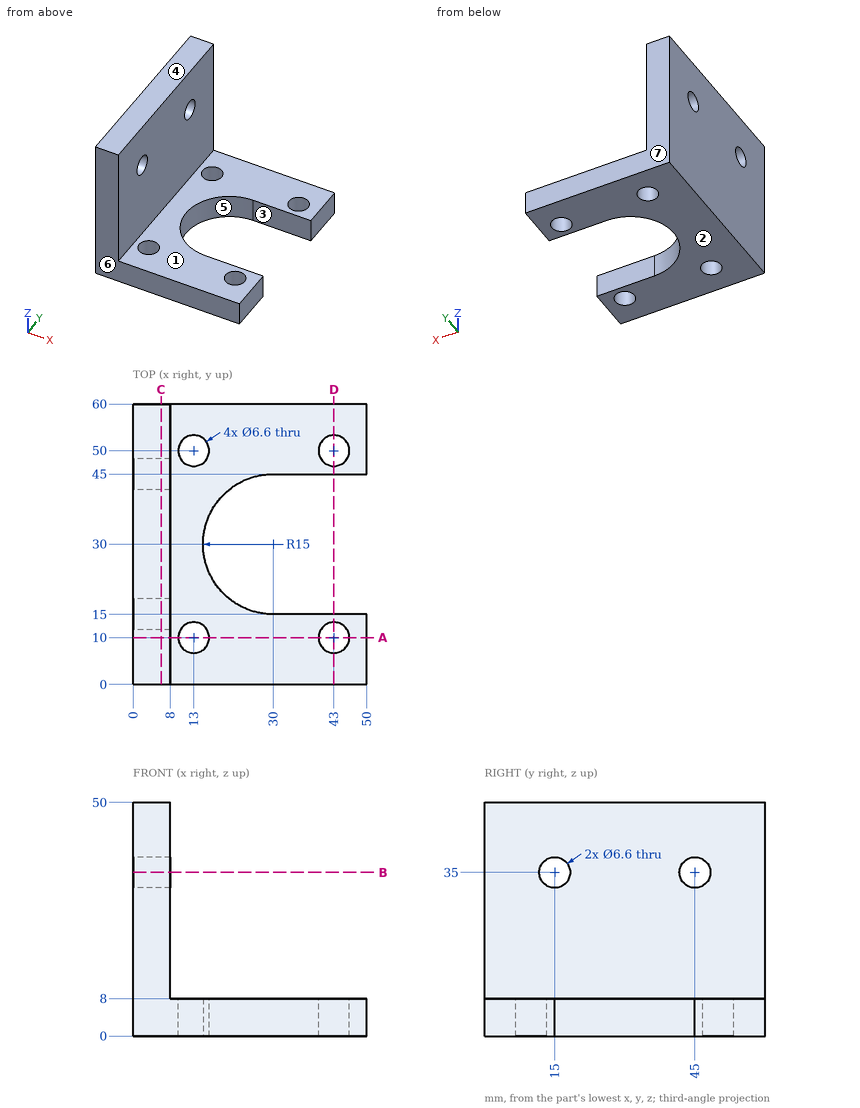
Can you work these out from the drawing? Everything is in mm from the part's minimum corner. A direction names the side the tool comes from. Round coordinates to 2 decimals unless told otherwise and drop trailing zeros. Order: outer loops, then holes, each group sorted by start corner. A loop starts at its lowest first (then second) coordinate and runs counter-clockwise, first axis right, second up. Notation, with made-up numbers: (89, 25.5) -> (129, 25.5) arc R26 ccw to (129, 58.5) -> close; hole circle Ø6 at (36, 42). An arc over 180 degrees is marked (long way). Return JSON: item names as keys, results as strings. Group by question number.
1. If we section it at C-C, the plane x = 6: Write out the boundary of the cut face in (y, z).
2. I need wall thicknesses on line 1 (Y direction, x = 13, z = 2.5); line 2 (X direction, y = 10, z = 3.75); line 3 (X direction, y = 8, z = 32.5). Which ranges of each line are inside material? Lowest first, please. Write a range as [from, to].
3. If we section it at D-D, the plane x = 43: Write out the boundary of the cut face in (y, z), then the cut area to 3 significant figures.
4. Will these pins go through, and if not, where does the flat tip stop? pin 1 (5 mm diameter, centred on y = 24.5, z = 6, fed in from +X); pin 2 (5.5 mm diameter, centred on y = 45, z = 35, fed in from -X); pin 3 (8.5 mm diameter, centred on y = 15, z = 35, fed in from +X); pin 4 (7.5 mm diameter, centred on x = 43, y = 50, fed in from +Z).
5. Which directions (+Z, -Z, +X, -X, +Y, -Y) give clear straight access to the entire face, cutting with the end or side of a thin tool? Please do the marked faces 1, 2 and 3.
6. If we section it at B-B, the plane z = 35: Write out the boundary of the cut face in (x, y).
7. If we section it at A-A, the plane y = 10: Write out the boundary of the cut face in (x, z), then the cut area to 3 significant figures.
8. We'd pull the mould along Y, two halves only. Please class the marked faces 4, 5, 6 and 7: released by +Y, released by -Y, zero draft, split by the parting line, or undercut.
Output values:
{
 "1": {"outline": "(0, 0) -> (60, 0) -> (60, 50) -> (0, 50) -> close; hole circle Ø6.6 at (15, 35); hole circle Ø6.6 at (45, 35)"},
 "2": {"line 1": "[0, 6.7], [13.3, 46.7], [53.3, 60]", "line 2": "[0, 9.7], [16.3, 39.7], [46.3, 50]", "line 3": "[0, 8]"},
 "3": {"outline": "(0, 0) -> (6.7, 0) -> (6.7, 8) -> (0, 8) -> close; (13.3, 0) -> (15, 0) -> (15, 8) -> (13.3, 8) -> close; (45, 0) -> (46.7, 0) -> (46.7, 8) -> (45, 8) -> close; (53.3, 0) -> (60, 0) -> (60, 8) -> (53.3, 8) -> close", "area": "134 mm²"},
 "4": {"pin 1": "x = 17.31", "pin 2": "through", "pin 3": "x = 8", "pin 4": "z = 8"},
 "5": {"face 1": "+Z, +X, +Y, -Y", "face 2": "-Z, +X, -X, +Y, -Y", "face 3": "+Z, -Z, +X"},
 "6": {"outline": "(0, 0) -> (8, 0) -> (8, 11.7) -> (0, 11.7) -> close; (0, 18.3) -> (8, 18.3) -> (8, 41.7) -> (0, 41.7) -> close; (0, 48.3) -> (8, 48.3) -> (8, 60) -> (0, 60) -> close"},
 "7": {"outline": "(0, 0) -> (9.7, 0) -> (9.7, 8) -> (8, 8) -> (8, 50) -> (0, 50) -> close; (16.3, 0) -> (39.7, 0) -> (39.7, 8) -> (16.3, 8) -> close; (46.3, 0) -> (50, 0) -> (50, 8) -> (46.3, 8) -> close", "area": "630 mm²"},
 "8": {"face 4": "zero draft", "face 5": "undercut", "face 6": "released by -Y", "face 7": "released by +Y"}
}
